from build123d import *

# Parameters (mm, degrees)
BOSS_EXTRUDE1_DEPTH = 1.59
SKETCH3_R           = 1.59
SKETCH3_R_2         = 0.51
CUT_EXTRUDE1_DEPTH  = 66.073251801


with BuildPart() as part:
    # Sketch1 → Boss-Extrude1 (new body)
    with BuildSketch(Plane(origin=(0, 0, 0), x_dir=(1, 0, 0), z_dir=(0, 1, 0))):
        Polygon((-38, 46), (-46, 38), (-46, -38), (-38, -46), (38, -46), (46, -38), (46, 38), (38, 46), align=None)
    extrude(amount=BOSS_EXTRUDE1_DEPTH)

    # Sketch3 → Cut-Extrude1 (cut, through all)
    with BuildSketch(Plane(origin=(0, 1.59, 0), x_dir=(1, 0, 0), z_dir=(0, 1, 0))):
        with Locations(Location((-39.5, 39.5, 0), (0, 0, 270))):
            Circle(SKETCH3_R)
        with Locations(Location((39.5, 39.5, 0), (0, 0, 270))):
            Circle(SKETCH3_R)
        with Locations(Location((39.5, -39.5, 0), (0, 0, 270))):
            Circle(SKETCH3_R)
        with Locations(Location((-39.5, -39.5, 0), (0, 0, 270))):
            Circle(SKETCH3_R)
        with Locations(Location((-2.67, -21.93, 0), (0, 0, 270))):
            Circle(SKETCH3_R_2)
        with Locations(Location((2.03, -22.75, 0), (0, 0, 270))):
            Circle(SKETCH3_R_2)
        with Locations(Location((-2.67, -42.07, 0), (0, 0, 270))):
            Circle(SKETCH3_R_2)
        with Locations(Location((2.03, -41.24, 0), (0, 0, 270))):
            Circle(SKETCH3_R_2)
    extrude(amount=-CUT_EXTRUDE1_DEPTH, mode=Mode.SUBTRACT)


solid = part.part
Verification items for the finished model (mm, model axes). Coordinates: 2 decimals unless noted, no trailing zeros. Loops run counter-clockwise (first coordinate to the right, second up) from the corner with the lowest first, then second, coordinate; pieces in that order, holes last. Notation, with made-up numbers: (-25, 86.5) -> (-5, 86.5) arc R27 cw to (-5, 104.5) -> close; hole circle Ø3 at (58, 52). An arc over 180 degrees is marked (long way). Answer as CSV lines item,"result".
1) Thickness scan on L1, parallel to X at y = 1.3, z = 22.75; L2, parallel to X at y = 0.5, z = -39.5; L3, parallel to X at y = 1.1, z = -41.5. Record the ranges inside material, lowest first. Write a range as from..to.
Found:
L1,"x = -46..1.52, 2.54..46"
L2,"x = -44.5..-41.09, -37.91..37.91, 41.09..44.5"
L3,"x = -42.5..42.5"
2) Depth check by flat-ended pin: pin 1 (0.6 mm diameter, centred on x = -2.67, z = 21.93, fed in from +Y). Enter the tip coordinate at first touch or a pass-through.
Found:
pin 1,"passes through"
3) Release check for a two-part mould opening along X. For faces 1 (the cylindrical face through (39.978, 0.806, -37.983)), 2 (the flat face through (42, 1, 42)), 3 (the flat face through (-42, 1, -42)) record: +X half, -X half, draft (parallel to the pull), parting line (faces both ways), or undercut.
Found:
face 1,"undercut"
face 2,"+X half"
face 3,"-X half"
4) Cross-section at B-B, the plane x = 39.5. Record the cut outline in (y, z), then the cut area to 3 significant figures.
Found:
outline,"(0, -44.5) -> (1.59, -44.5) -> (1.59, -41.09) -> (0, -41.09) -> close; (0, -37.91) -> (1.59, -37.91) -> (1.59, 37.91) -> (0, 37.91) -> close; (0, 41.09) -> (1.59, 41.09) -> (1.59, 44.5) -> (0, 44.5) -> close"
area,"131 mm2"
5) Cross-section at A-A, the plane y = 1.1. Count the separate pieces of the cut face and the enclosed holes in it, then the cut area to 3 significant figures.
Found:
separate pieces,"1"
enclosed holes,"8"
area,"8,300 mm2"
